```python
from build123d import *

# Parameters (mm, degrees)
CROQUIS1_W              = 65
CROQUIS1_H              = 95
SALIENTE_EXTRUIR1_DEPTH = 2.5
CROQUIS3_R              = 1.5
CORTAR_EXTRUIR2_DEPTH   = 58.608593109
CROQUIS4_R              = 20
CORTAR_EXTRUIR3_DEPTH   = 58.608593109


with BuildPart() as part:
    # Croquis1 → Saliente-Extruir1 (new body)
    with BuildSketch(Plane(origin=(0, 0, 0), x_dir=(1, 0, 0), z_dir=(0, 1, 0))):
        Rectangle(CROQUIS1_W, CROQUIS1_H)
    extrude(amount=SALIENTE_EXTRUIR1_DEPTH)

    # Croquis3 → Cortar-Extruir2 (cut, through all)
    with BuildSketch(Plane(origin=(0, 2.5, 0), x_dir=(1, 0, 0), z_dir=(0, 1, 0))):
        with Locations(Location((27.5, 42.5, 0), (0, 0, 270))):
            Circle(CROQUIS3_R)
        with Locations(Location((7.5, 32.5, 0), (0, 0, 270))):
            Circle(CROQUIS3_R)
        with Locations(Location((7.5, -32.5, 0), (0, 0, 90))):
            Circle(CROQUIS3_R)
        with Locations(Location((27.5, -42.5, 0), (0, 0, 90))):
            Circle(CROQUIS3_R)
        with Locations(Location((-27.5, 42.5, 0), (0, 0, 90))):
            Circle(CROQUIS3_R)
        with Locations(Location((-7.5, 32.5, 0), (0, 0, 90))):
            Circle(CROQUIS3_R)
        with Locations(Location((-27.5, -42.5, 0), (0, 0, 270))):
            Circle(CROQUIS3_R)
        with Locations(Location((-7.5, -32.5, 0), (0, 0, 270))):
            Circle(CROQUIS3_R)
    extrude(amount=-CORTAR_EXTRUIR2_DEPTH, mode=Mode.SUBTRACT)

    # Croquis4 → Cortar-Extruir3 (cut, through all)
    with BuildSketch(Plane(origin=(0, 2.5, 0), x_dir=(1, 0, 0), z_dir=(0, 1, 0))):
        with Locations(Location((0, 0, 0), (0, 0, 270))):
            Circle(CROQUIS4_R)
    extrude(amount=-CORTAR_EXTRUIR3_DEPTH, mode=Mode.SUBTRACT)


solid = part.part
```
Design review of the part built by this model. Coordinates are the model's own, in mm. Coordinates: 2 decimals unless noted, no trailing zeros. Loops run counter-clockwise (first coordinate to the right, second up) from the corner with the lowest first, then second, coordinate; pieces in that order, holes last. Notation, with made-up numbers: (-23.5, 86.5) -> (15.5, 86.5) arc R14 ccw to (15.5, 103.5) -> close; hole circle Ø10 at (18.25, 62.5). An arc over 180 degrees is marked (long way). Answer as a JSON object with one key per item and string values.
Q1. Take a section at C-C on y = 2. Give the number of separate pieces and of enclosed holes in the cut face, plus the area to 3 significant figures.
Answer block:
{"separate pieces": "1", "enclosed holes": "9", "area": "4,860 mm^2"}
Q2. The part is to be moulded in two halves that separate along X. For faces 1 (the flat face through (-0.5, 0, 20.4)), 2 (the flat face through (32.5, 1, 1)), 3 (the flat face through (-32.5, 1, 1)), 4 (the cylindrical face through (-8.4, 1.3, 31.3)), say which applies: +X half, -X half, draft (parallel to the pull), parting line (faces both ways), or undercut.
Answer block:
{"face 1": "draft", "face 2": "+X half", "face 3": "-X half", "face 4": "undercut"}
Q3. To check wall thickness, follow L1, parallel to X at y = 1.3, z = 42.5; L2, parallel to X at y = 1.45, z = 32.5; L3, parallel to Z at x = 7, y = 1.2 (3 decimals). State the ranges of each line that lie inside material, in increasing order.
Answer block:
{"L1": "x = -32.5 to -29, -26 to 26, 29 to 32.5", "L2": "x = -32.5 to -9, -6 to 6, 9 to 32.5", "L3": "z = -47.5 to -33.914, -31.086 to -18.735, 18.735 to 31.086, 33.914 to 47.5"}
Q4. Take a section at A-A on x = 0. Give the boundary of the cut face in (y, z).
Answer block:
{"outline": "(0, -47.5) -> (2.5, -47.5) -> (2.5, -20) -> (0, -20) -> close; (0, 20) -> (2.5, 20) -> (2.5, 47.5) -> (0, 47.5) -> close"}
Q5. Take a section at D-D on z = 42.5. Give the boundary of the cut face in (x, y), plus the area to 4 significant figures.
Answer block:
{"outline": "(-32.5, 0) -> (-29, 0) -> (-29, 2.5) -> (-32.5, 2.5) -> close; (-26, 0) -> (26, 0) -> (26, 2.5) -> (-26, 2.5) -> close; (29, 0) -> (32.5, 0) -> (32.5, 2.5) -> (29, 2.5) -> close", "area": "147.5 mm^2"}
Q6. Take a section at B-B on z = 0. Give the boundary of the cut face in (x, y), plus the area to 3 significant figures.
Answer block:
{"outline": "(-32.5, 0) -> (-20, 0) -> (-20, 2.5) -> (-32.5, 2.5) -> close; (20, 0) -> (32.5, 0) -> (32.5, 2.5) -> (20, 2.5) -> close", "area": "62.5 mm^2"}
